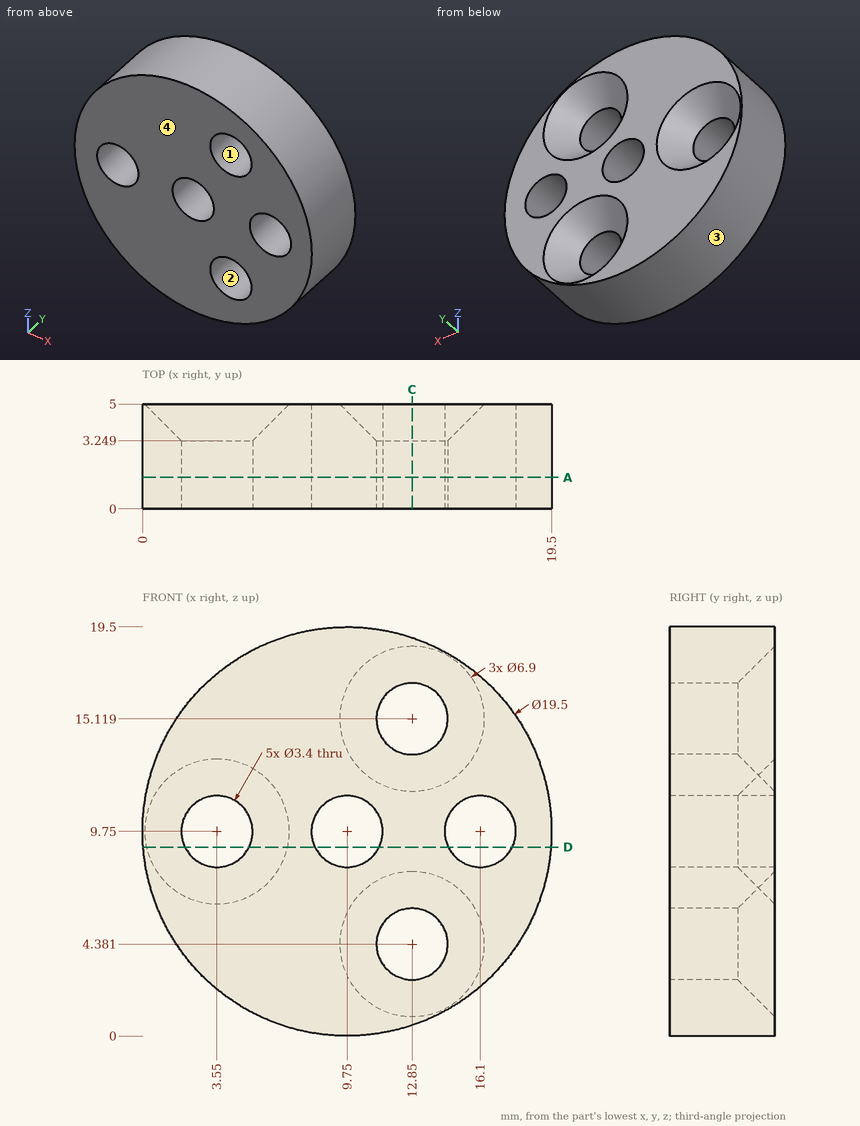
Design review of the part shown in the three views and the two pictorial views. Dimensions are in mm from the part's minimum x, y and z. Round coordinates to 2 decimals unless told otherwise and drop trailing zeros. Order: outer loops, then holes, each group sorted by start corner. A loop starts at its lowest first (then second) coordinate and runs counter-clockwise, first axis right, second up.
(1) Take a section at D-D, the plane z = 9. Count the separate pieces of the cut face and the enclosed holes in it.
Working result:
separate pieces: 4
enclosed holes: 0
(2) Take a section at A-A, the plane y = 1.5. State the section outline as (x, z) points, plus the area to 3 significant figures.
Working result:
outline: circle Ø19.5 at (9.75, 9.75); hole circle Ø3.4 at (3.55, 9.75); hole circle Ø3.4 at (9.75, 9.75); hole circle Ø3.4 at (12.85, 4.38); hole circle Ø3.4 at (12.85, 15.12); hole circle Ø3.4 at (16.1, 9.75)
area: 253 mm2
(3) Take a section at C-C, the plane x = 12.85. State the section outline as (y, z) points.
Working result:
outline: (0, 0.51) - (5, 0.51) - (5, 0.93) - (3.25, 2.68) - (0, 2.68) - close; (0, 6.08) - (3.25, 6.08) - (5, 7.83) - (5, 11.67) - (3.25, 13.42) - (0, 13.42) - close; (0, 16.82) - (3.25, 16.82) - (5, 18.57) - (5, 18.99) - (0, 18.99) - close
(4) Mouldability with a two-part tool opening along Z and no side actions: class the marked faces 1, 2, 3 and 4 as released by +Z, released by -Z, zero draft, split by the parting line, or undercut.
Working result:
face 1: undercut
face 2: undercut
face 3: split by the parting line
face 4: zero draft
(5) For P1, Ø1, axis at y = 0.5, z = 11, coming from the +X side; P2, Ø5.5, axis at x = 12.85, z = 15.12, coming from the +Y side; P3, Ø3, axis at x = 16.1, z = 9.75, coming from the +Y side, all flat-tipped, find the tip position at first contact; note any pin that passes through.
Working result:
P1: stops at x = 19.47
P2: stops at y = 4.3
P3: passes through
(6) Wall thickness on L1, parallel to Z at x = 9.75, y = 2.3; L2, parallel to X at y = 3.05, z = 10.5 (1 decimal); L3, parallel to Z at x = 12.85, y = 1.15 (1 decimal): over which ranges is each line inside the solid? List them lowest first.
Working result:
L1: z = 0 to 8.05, 11.45 to 19.5
L2: x = 0 to 2, 5.1 to 8.2, 11.3 to 14.6, 17.6 to 19.5
L3: z = 0.5 to 2.7, 6.1 to 13.4, 16.8 to 19
